from build123d import *

# Parameters (mm, degrees)
F0_W     = 40
F0_H     = 40
F1_DEPTH = 20
F2_R     = 5.08
F3_D     = 25.4
F3_DEPTH = 20.001


with BuildPart() as f1:
    # F0 (on Top) → F1 (new body, symmetric)
    with BuildSketch(Plane.XY):
        Rectangle(F0_W, F0_H)
    extrude(amount=F1_DEPTH, both=True)

    # F2
    f2_edges = [f1.edges().sort_by_distance(p)[0] for p in [
        (0, -20, 20),
        (20, 0, 20),
        (0, 20, 20),
        (-20, 0, 20),
        (-20, -20, 0),
        (20, -20, 0),
        (20, 0, -20),
        (20, 20, 0),
        (0, -20, -20),
        (-20, 0, -20),
        (0, 20, -20),
        (-20, 20, 0),
    ]]
    fillet(f2_edges, radius=F2_R)

    # F3 (through all, one way)
    with BuildSketch(Plane(origin=(0, 0, 0), x_dir=(1, 0, 0), z_dir=(0, 0, -1))):
        with Locations((0, 0)):
            Circle(F3_D / 2)
    extrude(amount=-F3_DEPTH, mode=Mode.SUBTRACT)


solid = f1.part
Verification items for the finished model (mm, model axes). A direction names the side the tool comes from. Give positions to 0.01 mm unless a question says otherwise; leave off trailing zeros. Write each loop counter-clockwise with the first axis right and the second up, starting at its lowest first coordinate (ties: lowest second). Pieces come first, ordered by that corner, then holes. Notation, with made-up numbers: (9, 86.5) - (48, 86.5) arc R33 ccw to (48, 115.5) - close; hole circle Ø2 at (1, -3.75). An arc over 180 degrees is marked (long way). Answer as CSV lines item,"result". Start each with the question number.
1. Sectioned sample at A-A (z = 9). Record the boundary of the cut face in (x, y), then the cut area to 3 significant figures.
2. Thickness scan on line 1 (X direction, y = 0, z = 11.75); line 2 (Z direction, x = 3, y = -7.5). Record the ranges inside material, lowest first.
3. Depth check by flat-ended pin: pin 1 (1 mm diameter, centred on x = 5.5, y = 5.5, fed in from +Z). Enter the tip coordinate at first touch or a pass-through.
4. Draft check along X on faces 3 (the face through (0, 0, 0)), 4 (the face through (0.209, 18.551, -18.472)), 5 (the face through (18.551, 0.209, -18.472)). Enter one of: pulls with the +X half, pulls with the -X half, needs draft (parallel to the pull), parting line crosses it, or undercut.
5. Set-up check for faces 1 (the face through (-2.75, 12.4, 9.86)), 2 (the face through (18.551, -18.472, 0.209)): record each of +Z, -Z, +X, -X, +Y, -Y from which the full face is reachable in a straight line by a thin tool's end or side.
6. Sectioned sample at B-B (x = 0). Record the boundary of the cut face in (y, z).
Derived:
1,outline,"(-20, -14.92) arc R5.08 ccw to (-14.92, -20) - (14.92, -20) arc R5.08 ccw to (20, -14.92) - (20, 14.92) arc R5.08 ccw to (14.92, 20) - (-14.92, 20) arc R5.08 ccw to (-20, 14.92) - close; hole circle Ø25.4 at (0, 0)"
1,area,"1,070 mm²"
2,line 1,"-20 to -12.7, 12.7 to 20"
2,line 2,"-20 to 0"
3,pin 1,"z = 0"
4,face 3,"undercut"
4,face 4,"needs draft"
4,face 5,"pulls with the +X half"
5,face 1,"+Z"
5,face 2,"+Z, -Z, +X, -Y"
6,outline,"(-20, -14.92) arc R5.08 ccw to (-14.92, -20) - (14.92, -20) arc R5.08 ccw to (20, -14.92) - (20, 14.92) arc R5.08 ccw to (14.92, 20) - (12.7, 20) - (12.7, 0) - (-12.7, 0) - (-12.7, 20) - (-14.92, 20) arc R5.08 ccw to (-20, 14.92) - close"
